The drawing under review shows one solid part. Ordinate dimensions are in mm from its lowest x, y, z. A direction names the side the tool comes from. Coordinates: 2 decimals unless noted, no trailing zeros. Write each loop counter-clockwise with the first axis right and the second up, starting at its lowest first coordinate (ties: lowest second). Pieces come first, ordered by that corner, then holes.
Q1. Take a section at A-A (x = 20). Give the boundary of the cut face in (y, z) (1 decimal).
Q2. For probe 1 along Z at (x, y) = (2.5, 45) (1 decimal); probe 2 along X at (y, z) = (35, 17); probe 3 along Z at (x, y) = (28, 53) (1 decimal), list the stretches that pass through material, from the lowest coordinate up.
Q3. Mouldability with a two-part tool opening along Z and no side actions: class the marked faces 3, 4 and 5 as pulls with the +Z half, pulls with the -Z half, needs draft (parallel to the pull), parting line crosses it, or undercut.
Q4. Take a section at D-D (x = 11). Give the boundary of the cut face in (y, z) (1 decimal).
Q5. Take a section at B-B (y = 12.7). State how many separate pieces and enclosed holes the cut face has.
Q6. Machinability: for the marked faces 1 and 2, which of the approach directions +Z, -Z, +X, -X, +Y, -Y give a long, thin tool a straight path to every point of the face, cutting with its end or side? Answer none if there is none.
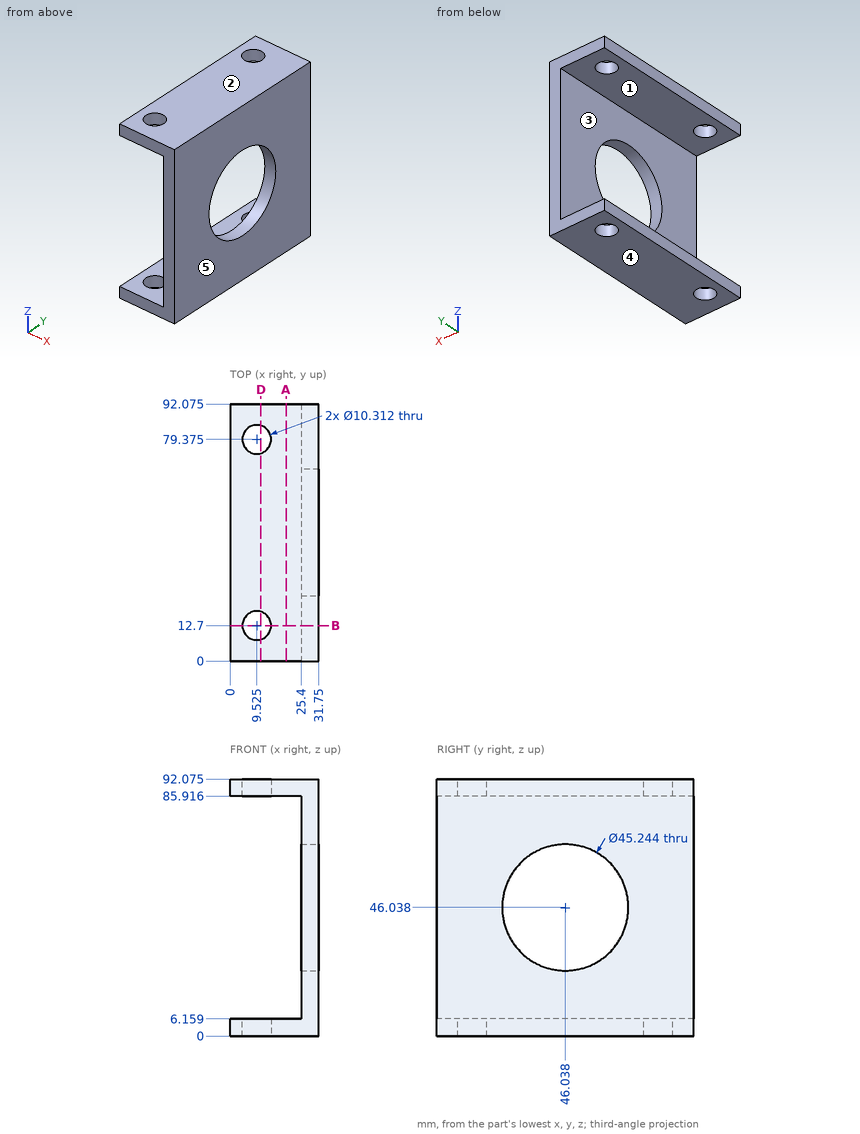
Response:
1. outline: (0, 0) - (92.1, 0) - (92.1, 6.2) - (0, 6.2) - close; (0, 85.9) - (92.1, 85.9) - (92.1, 92.1) - (0, 92.1) - close
2. probe 1: z = 0 to 6.2, 85.9 to 92.1
2. probe 2: x = 25.4 to 31.75
2. probe 3: z = 0 to 24.5, 67.6 to 92.1
3. face 3: undercut
3. face 4: pulls with the -Z half
3. face 5: needs draft
4. outline: (0, 0) - (7.8, 0) - (7.8, 6.2) - (0, 6.2) - close; (0, 85.9) - (7.8, 85.9) - (7.8, 92.1) - (0, 92.1) - close; (17.6, 0) - (74.4, 0) - (74.4, 6.2) - (17.6, 6.2) - close; (17.6, 85.9) - (74.4, 85.9) - (74.4, 92.1) - (17.6, 92.1) - close; (84.3, 0) - (92.1, 0) - (92.1, 6.2) - (84.3, 6.2) - close; (84.3, 85.9) - (92.1, 85.9) - (92.1, 92.1) - (84.3, 92.1) - close
5. separate pieces: 3
5. enclosed holes: 0
6. face 1: -X, +Y, -Y
6. face 2: +Z, +X, -X, +Y, -Y
